Input: part model. Units: mm. Frame: model coordinates. A direction names the side the tool comes from. Round coordinates to 2 decimals unless told otherwise and drop trailing zeros. Order: outer loops, then holes, each group sorted by start corner. A loop starts at its lowest first (then second) coordinate and runs counter-clockwise, first axis right, second up.
Item 1: Cut plane D-D on x = 2.5. Output: boundary loops of the cut face in (y, z).
Item 2: First-contact query: pin 1 (1 mm diameter, centred on x = 2.5, z = -28.5, fed in from +Y). Flat tip, straight axial feed; report the tip coordinate or a pass-through.
Item 3: Cut plane C-C on y = 21. Output: boundary loops of the cut face in (x, z), then the cut area to 3 significant figures.
Item 4: Cut plane A-A on z = -8. Output: boundary loops of the cut face in (x, y), then the cut area to 3 significant figures.
Item 5: Mould query, pull axis X, two halves, no side actions, for faces 1 (the flat face through (0, 26.5, 39)), 2 (the cylindrical face through (6.23, 0.74, -7.03)), 3 (the flat face through (-10, 1, 12)). Classes: released by +X, released by -X, zero draft, split by the parting line, or undercut.
Item 6: Line query: L1, parallel to X at y = 0.6, z = -8; L2, parallel to Z at x = 5.75, y = 5.75; L3, parallel to Z at x = -7.5, y = 0.7. Output: solid intervals per line, ascending.
Item 7: Cut plane B-B on x = -7.5. Output: boundary loops of the cut face in (y, z), then the cut area to 3 significant figures.
Item 8: Reachability of faces 4 (the cylindrical face through (7.15, 0.74, 9.56)), 5 (the flat face through (0, 1.5, -1)) from +Z, -Z, +X, -X, +Y, -Y: full face, straight path, thin tool, end or side. Return the list, or none.
```python
from build123d import *

# Parameters (mm, degrees)
SKETCH2_W           = 20
SKETCH2_H           = 80
SKETCH2_R           = 1.6
BOSS_EXTRUDE1_DEPTH = 1.5
SKETCH3_W           = 20
SKETCH3_H           = 1.5
BOSS_EXTRUDE2_DEPTH = 25
FILLET1_R           = 1
FILLET2_R           = 2.5


with BuildPart() as part:
    # Sketch2 → Boss-Extrude1 (new body)
    with BuildSketch(Plane(origin=(0, 0, 0), x_dir=(1, 0, 0), z_dir=(0, 1, 0))):
        Rectangle(SKETCH2_W, SKETCH2_H)
        with Locations((-7.5, 8)):
            Circle(SKETCH2_R, mode=Mode.SUBTRACT)
        with Locations((7.5, 8)):
            Circle(SKETCH2_R, mode=Mode.SUBTRACT)
        with Locations((-7.5, -8)):
            Circle(SKETCH2_R, mode=Mode.SUBTRACT)
        with Locations((7.5, -8)):
            Circle(SKETCH2_R, mode=Mode.SUBTRACT)
    extrude(amount=BOSS_EXTRUDE1_DEPTH)

    # Sketch3 → Boss-Extrude2 (add)
    with BuildSketch(Plane(origin=(0, 1.5, 0), x_dir=(1, 0, 0), z_dir=(0, 1, 0))):
        with Locations((0, 39.25)):
            Rectangle(SKETCH3_W, SKETCH3_H)
        with Locations((0, -39.25)):
            Rectangle(SKETCH3_W, SKETCH3_H)
    extrude(amount=BOSS_EXTRUDE2_DEPTH)

    # Fillet1
    fillet1_edges = [part.edges().sort_by_distance(p)[0] for p in [
        (0, 1.5, -38.5),
        (0, 1.5, 38.5),
    ]]
    fillet(fillet1_edges, radius=FILLET1_R)

    # Fillet2
    fillet2_edges = [part.edges().sort_by_distance(p)[0] for p in [
        (0, 0, 40),
        (0, 0, -40),
    ]]
    fillet(fillet2_edges, radius=FILLET2_R)


solid = part.part
```
From the geometry:
1. outline: (0, -37.5) arc R2.5 ccw to (2.5, -40) - (26.5, -40) - (26.5, -38.5) - (2.5, -38.5) arc R1 cw to (1.5, -37.5) - (1.5, 37.5) arc R1 cw to (2.5, 38.5) - (26.5, 38.5) - (26.5, 40) - (2.5, 40) arc R2.5 ccw to (0, 37.5) - close
2. pin 1: stops at y = 1.5
3. outline: (-10, -40) - (10, -40) - (10, -38.5) - (-10, -38.5) - close; (-10, 38.5) - (10, 38.5) - (10, 40) - (-10, 40) - close
3. area: 60.0 mm2
4. outline: (-10, 0) - (-9.1, 0) - (-9.1, 1.5) - (-10, 1.5) - close; (-5.9, 0) - (5.9, 0) - (5.9, 1.5) - (-5.9, 1.5) - close; (9.1, 0) - (10, 0) - (10, 1.5) - (9.1, 1.5) - close
4. area: 20.4 mm2
5. face 1: zero draft
5. face 2: undercut
5. face 3: released by -X
6. L1: x = -10 to -9.1, -5.9 to 5.9, 9.1 to 10
6. L2: z = -40 to -38.5, 38.5 to 40
6. L3: z = -39.23 to -9.6, -6.4 to 6.4, 9.6 to 39.23
7. outline: (0, -37.5) arc R2.5 ccw to (2.5, -40) - (26.5, -40) - (26.5, -38.5) - (2.5, -38.5) arc R1 cw to (1.5, -37.5) - (1.5, -9.6) - (0, -9.6) - close; (0, -6.4) - (1.5, -6.4) - (1.5, 6.4) - (0, 6.4) - close; (0, 9.6) - (1.5, 9.6) - (1.5, 37.5) arc R1 cw to (2.5, 38.5) - (26.5, 38.5) - (26.5, 40) - (2.5, 40) arc R2.5 ccw to (0, 37.5) - close
7. area: 183 mm2
8. face 4: +Y, -Y
8. face 5: +X, -X, +Y
